```python
from build123d import *

# Parameters (mm, degrees)
SKETCH2_R         = 10
EXTRUDE1_DEPTH    = 200
EXTRUDE2_DEPTH    = 30
SKETCH5_OUTSIDE_W = 62.398
SKETCH5_OUTSIDE_H = 62.398
SKETCH5_OUTSIDE_R = 7.5
EXTRUDE4_DEPTH    = 140
SKETCH6_R         = 11
SKETCH6_R_2       = 8.630699516
EXTRUDE5_DEPTH    = 5
SKETCH7_W         = 11.867066039
SKETCH7_H         = 33.623353778
EXTRUDE6_DEPTH    = 20


with BuildPart() as part:
    # Sketch2 → Extrude1 (new body)
    with BuildSketch(Plane(origin=(0, 0, 0), x_dir=(1, 0, 0), z_dir=(0, 1, 0))):
        with Locations(Location((0, 0, 0), (0, 0, 270))):
            Circle(SKETCH2_R)
    extrude(amount=EXTRUDE1_DEPTH)

    # Sketch3 → Extrude2 (cut)
    with BuildSketch(Plane(origin=(0, 200, 0), x_dir=(1, 0, 0), z_dir=(0, 1, 0))):
        with BuildLine():
            Line((2, 5.656854249), (2, 7.749317393))
            Line((2, 7.749317393), (-2, 7.749317393))
            Line((-2, 7.749317393), (-2, 5.656854249))
            ThreePointArc((-2, 5.656854249), (0, -6), (2, 5.656854249))
        make_face()
    extrude(amount=-EXTRUDE2_DEPTH, mode=Mode.SUBTRACT)

    # Sketch5 outside → Extrude4 (cut)
    with BuildSketch(Plane.XZ):
        Rectangle(SKETCH5_OUTSIDE_W, SKETCH5_OUTSIDE_H)
        with Locations(Location((0, 0, 0), (0, 0, 270))):
            Circle(SKETCH5_OUTSIDE_R, mode=Mode.SUBTRACT)
    extrude(amount=-EXTRUDE4_DEPTH, mode=Mode.SUBTRACT)

    # Sketch6 → Extrude5 (add)
    with BuildSketch(Plane(origin=(0, 200, 0), x_dir=(1, 0, 0), z_dir=(0, 1, 0))):
        with Locations(Location((0, 0, 0), (0, 0, 270))):
            Circle(SKETCH6_R)
        Circle(SKETCH6_R_2, mode=Mode.SUBTRACT)
    extrude(amount=-EXTRUDE5_DEPTH)

    # Sketch7 → Extrude6 (cut)
    with BuildSketch(Plane.XZ):
        with Locations((11.93353302, 6.659772738)):
            Rectangle(SKETCH7_W, SKETCH7_H)
    extrude(amount=-EXTRUDE6_DEPTH, mode=Mode.SUBTRACT)


solid = part.part
```
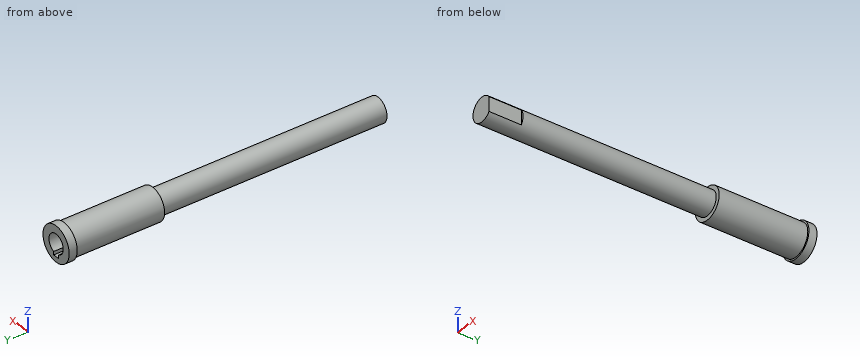
Input: part model. Units: mm. Frame: model coordinates. Round coordinates to 2 decimals unless told otherwise and drop trailing zeros. Write each loop counter-clockwise with the first axis right and the second up, starting at its lowest first coordinate (ties: lowest second). Pieces come first, ordered by that corner, then holes. Notation, with made-up numbers: (-39, -21.75) -> (-8, -21.75) arc R13 cw to (-8, -4.75) -> close; hole circle Ø6 at (18, 25). An arc over 180 degrees is marked (long way). Answer as CSV lines item,"result".
1. Ray query, L1, parallel to Z at x = 0, y = 179.25; L2, parallel to X at y = 184, z = 0; L3, parallel to Y at x = 3.25, z = -3.25. Return the intervals inside material, ascending. Write a range as [from, to].
Geometry says:
L1,"z = [-10, -7.75], [6, 10]"
L2,"x = [-10, -6], [6, 10]"
L3,"y = [0, 170]"
2. Section C-C (y = 70). Return the cut outline in (x, z).
Geometry says:
outline,"circle Ø15 at (0, 0)"
3. Section A-A (z = 0). Return the cut outline in (x, y), plus the area to 3 significant figures.
Geometry says:
outline,"(-11, 195) -> (-10, 195) -> (-10, 140) -> (-7.5, 140) -> (-7.5, 0) -> (6, 0) -> (6, 20) -> (7.5, 20) -> (7.5, 140) -> (10, 140) -> (10, 195) -> (11, 195) -> (11, 200) -> (6, 200) -> (6, 170) -> (-6, 170) -> (-6, 200) -> (-11, 200) -> close"
area,"2,920 mm^2"
4. Contact query for flat-ended pins moving along their axis: P1, Ø6, axis at y = 21.5, z = 5, coming from the +X side; P2, Ø1.5, axis at x = 3, z = 5, coming from the +Y side; P3, Ø7, axis at y = 8.5, z = 0.5, coming from the +X side; P4, Ø0.7, axis at x = 6.5, z = 0.5, coming from the -Y side. Output: stop coordinate, or through.
Geometry says:
P1,"stops at x = 7.23"
P2,"stops at y = 200"
P3,"stops at x = 6"
P4,"stops at y = 20"
5. Section B-B (x = 0). Return the cut outline in (y, z), plus the area to 3 significant figures.
Geometry says:
outline,"(0, -7.5) -> (140, -7.5) -> (140, -10) -> (195, -10) -> (195, -11) -> (200, -11) -> (200, -7.75) -> (170, -7.75) -> (170, 6) -> (200, 6) -> (200, 11) -> (195, 11) -> (195, 10) -> (140, 10) -> (140, 7.5) -> (0, 7.5) -> close"
area,"2,900 mm^2"
